```python
from build123d import *

# Parameters (mm, degrees)
F0_R     = 1.5875
F1_DEPTH = 3.048


with BuildPart() as f1:
    # F0 (on Front) → F1 (new body)
    with BuildSketch(Plane.XZ):
        with BuildLine():
            ThreePointArc((15.794203, 61.90038), (0, 47.625), (-15.794203, 61.90038))
            Line((-15.794203, 61.90038), (-9.525, 0))
            ThreePointArc((-9.525, 0), (0, 9.525), (9.525, 0))
            ThreePointArc((9.525, 0), (6.854788, -6.613434), (0.341271, -9.518884))
            Line((0.341271, -9.518884), (44.45, -7.9375))
            ThreePointArc((44.45, -7.9375), (36.5125, 0), (44.45, 7.9375))
            Line((44.45, 7.9375), (18.932251, 8.852361))
            ThreePointArc((18.932251, 8.852361), (13.224458, 11.573096), (11.307362, 17.598546))
            Line((11.307362, 17.598546), (15.794203, 61.90038))
        make_face()
        with BuildLine():
            Line((15.747457, 65.508289), (9.525, 114.3))
            ThreePointArc((9.525, 114.3), (0, 104.775), (-9.525, 114.3))
            Line((-9.525, 114.3), (-15.747457, 65.508289))
            ThreePointArc((-15.747457, 65.508289), (0, 79.375), (15.747457, 65.508289))
        make_face()
        with Locations((-3.175, 99.886943)):
            Circle(F0_R, mode=Mode.SUBTRACT)
        with BuildLine():
            ThreePointArc((15.875, 63.5), (15.843082, 64.506168), (15.747457, 65.508289))
            ThreePointArc((15.747457, 65.508289), (0, 79.375), (-15.747457, 65.508289))
            ThreePointArc((-15.747457, 65.508289), (-15.873668, 63.705667), (-15.794203, 61.90038))
            ThreePointArc((-15.794203, 61.90038), (0, 47.625), (15.794203, 61.90038))
            ThreePointArc((15.794203, 61.90038), (15.854788, 62.699171), (15.875, 63.5))
        make_face()
        with Locations((0, 63.5)):
            Circle(F0_R, mode=Mode.SUBTRACT)
        with BuildLine():
            ThreePointArc((-9.525, 114.3), (0, 104.775), (9.525, 114.3))
            ThreePointArc((9.525, 114.3), (0, 123.825), (-9.525, 114.3))
        make_face()
        with Locations((0, 114.3)):
            Circle(F0_R, mode=Mode.SUBTRACT)
        with BuildLine():
            ThreePointArc((9.525, 0), (0, 9.525), (-9.525, 0))
            ThreePointArc((-9.525, 0), (-6.613434, -6.854788), (0.341271, -9.518884))
            ThreePointArc((0.341271, -9.518884), (6.854788, -6.613434), (9.525, 0))
        make_face()
        Circle(F0_R, mode=Mode.SUBTRACT)
        with BuildLine():
            ThreePointArc((44.45, 7.9375), (36.5125, 0), (44.45, -7.9375))
            ThreePointArc((44.45, -7.9375), (50.06266, -5.61266), (52.3875, 0))
            ThreePointArc((52.3875, 0), (50.06266, 5.61266), (44.45, 7.9375))
        make_face()
        with Locations((44.45, 0)):
            Circle(F0_R, mode=Mode.SUBTRACT)
    extrude(amount=F1_DEPTH)


solid = f1.part
```
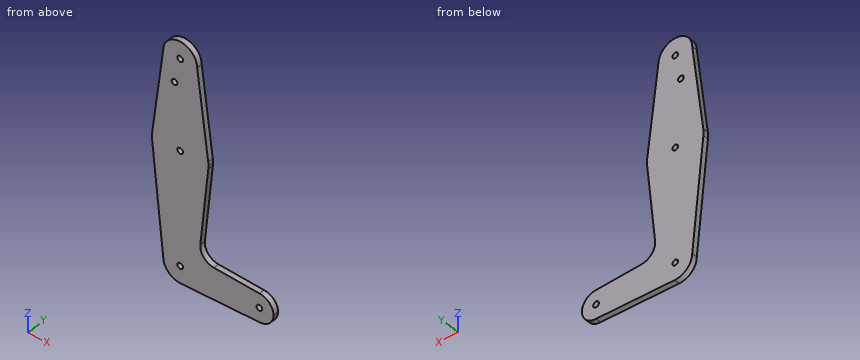
Part model, mm, in its own coordinate system. Give positions to 0.01 mm unless a question says otherwise; leave off trailing zeros. Order: outer loops, then holes, each group sorted by start corner. A loop starts at its lowest first (then second) coordinate and runs counter-clockwise, first axis right, second up. Notation, with made-up numbers: (-13.5, 36.25) - (25.5, 36.25) arc R11 ccw to (25.5, 43.25) - close; hole circle Ø3 at (6.5, 18). An arc over 180 degrees is marked (long way). Use one line per item in the form item = value.
Item 1: Pin check, flat tips, straight feed: pin 1 Ø2.5 at (x, z) = (0, 0) entering from -Y; pin 2 Ø1 at (y, z) = (-0.5, 100.5) entering from -X. Stop position of each tip, or through.
Solution:
pin_1 = through
pin_2 = -11.35
Item 2: Slice it at A-A on y = -0.6. Count the separate pieces of the cut face and the enclosed holes in it, and give its area (3 significant figures).
Solution:
separate_pieces = 1
enclosed_holes = 5
area = 3,890 mm2
Item 3: Probe probe 1 along Z at (x, y) = (0, -1.1) (1 decimal); probe 2 along X at (y, z) = (-0.95, 114.3) (1 decimal); probe 3 along X at (y, z) = (-0.15, 98.5). List the from-to ranges inside material, lowest first. Write a range as from..to.
Solution:
probe_1 = -9.5..-1.6, 1.6..61.9, 65.1..112.7, 115.9..123.8
probe_2 = -9.5..-1.6, 1.6..9.5
probe_3 = -11.54..-3.95, -2.4..11.54
Item 4: Slice it at B-B on z = 69.5. Give the cut face in (x, y), and give its area (3 significant figures).
Solution:
outline = (-15.24, -3.05) - (15.24, -3.05) - (15.24, 0) - (-15.24, 0) - close
area = 92.9 mm2
Item 5: Slice it at C-C on z = 109.5. Give the cut face in (x, y).
Solution:
outline = (-10.14, -3.05) - (10.14, -3.05) - (10.14, 0) - (-10.14, 0) - close
